Can you work these out from the model? Positions are in its coordinate system, mm. Face numbers are marked on the shaded views. A direction names the side the tool comes from. Coordinates: 2 decimals unless noted, no trailing zeros. Loops run counter-clockwise (first coordinate to the right, second up) from the corner with the lowest first, then second, coordinate; pieces in that order, holes last. Notation, with made-up numbers: (11.25, -24) -> (67.25, -24) arc R25 ccw to (67.25, 8) -> close; hole circle Ø1 at (-18.5, 48). An arc over 180 degrees is marked (long way). Use one line per item in the form item = value. Start each with the question number.
(1) Imagine slicing it at B-B (z = 385.5). List the corners of the cut face in (x, y) for me.
(2) I'm going to push flat-ended pins straight in: pin 1 (5 mm diameter, centred on x = 95.5, z = 207, fed in from -Y); pin 2 (5 mm diameter, centred on x = 414.5, y = -167, fed in from +Z); pin 3 (2 mm diameter, centred on y = -805, z = -1, fed in from -X). Where does each tip first touch, or does it pass through?
(3) Imagine slicing it at C-C (x = 127). List the corners of the cut face in (y, z) for me, plus the area to 3 significant figures.
(4) Imagine slicing it at D-D (x = 386). List the corners of the cut face in (y, z) for me, plus the area to 3 significant figures.
(5) I need wall thicknesses on line 1 (X direction, y = -793.5, z = 149); line 2 (Y direction, x = 472, z = 173); line 3 (Y direction, x = 45.5, z = 67.5). Which ranges of each line are inside material? Lowest first, please. Write a range as [from, to].
(6) On a 3-axis mill with a long thin cutter (end or side, diameter ignored), from which of +Z, -Z, +X, -X, +Y, -Y can I reach the whole of each face in a straight line? I mean the marked faces 5, 6 and 7. Say none if no direction works.
(7) Thinking about a two-plate mould opening in Y: for the marked faces 1, 2, 3 and 4, which applies, released by +Y, released by -Y, zero draft, split by the parting line, or undercut?
(8) Imagine slicing it at A-A (y = -231). List the corners of the cut face in (x, z) for me.
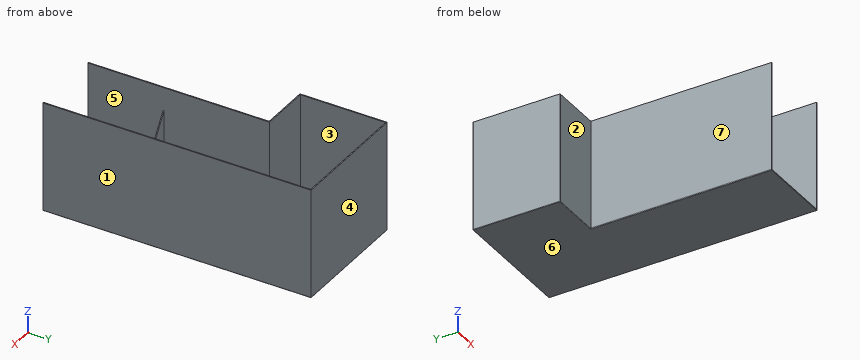
```python
from build123d import *

# Parameters (mm, degrees)
F1_DEPTH  = 426
F3_DEPTH  = 4
F4_R      = 2
F7_DEPTH  = 4
F8_DEPTH  = 4
F11_DEPTH = 4


# Not quite as in the source:
# - a feature names something its author has since deleted; it is built from what else it names


with BuildPart() as f1:
    # F0 (on Top) → F1 (new body)
    with BuildSketch(Plane.XY):
        Polygon((495, 0), (0, 0), (0, -343), (200, -343), (200, -1053), (204, -1053), (204, -339), (4, -339), (4, -4), (491, -4), (491, -1053), (495, -1053), align=None)
    extrude(amount=F1_DEPTH)

    # F2 (on Top) → F3 (join)
    with BuildSketch(Plane.XY):
        Polygon((0, -343), (200, -343), (199.9874711037, -1053), (495, -1053), (495, 0), (0, 0), align=None)
    extrude(amount=-F3_DEPTH)

    # F4
    f4_edges = [f1.edges().sort_by_distance(p)[0] for p in [
        (100, -343, -4),
        (0, -171.5, -4),
        (247.5, 0, -4),
        (0, -343, 211),
        (0, 0, 211),
        (495, 0, 211),
        (199.993736, -698, -4),
        (495, -526.5, -4),
    ]]
    fillet(f4_edges, radius=F4_R)

    # F6 (on offset) → F7 (join)
    with BuildSketch(Plane.XZ.offset(753)):
        Polygon((426, 0), (204, 335), (204, 0), align=None)
    extrude(amount=F7_DEPTH)

    # F6 (on offset) → F8 (join)
    with BuildSketch(Plane.XZ.offset(753)):
        Polygon((426, 0), (204, 335), (204, 0), align=None)
    extrude(amount=F8_DEPTH)

    # F10 (on offset) → F11 (join)
    with BuildSketch(Plane.XZ.offset(153)):
        Polygon((491, 335), (269, 0), (491, 0), align=None)
    extrude(amount=F11_DEPTH)


solid = f1.part
```
Worked out:
q1.outline = (0, -341) arc R2 ccw to (2, -343) -> (200, -343) -> (200, -1053) -> (204, -1053) -> (204, -339) -> (4, -339) -> (4, -4) -> (491, -4) -> (491, -1053) -> (495, -1053) -> (495, -2) arc R2 ccw to (493, 0) -> (2, 0) arc R2 ccw to (0, -2) -> close
q2.pin_1 = -343
q2.pin_2 = 0
q2.pin_3 = 199.99
q3.outline = (-343, -2) arc R2 ccw to (-341, -4) -> (-2, -4) arc R2 ccw to (0, -2) -> (0, 426) -> (-4, 426) -> (-4, 0) -> (-339, 0) -> (-339, 426) -> (-343, 426) -> close
q3.area = 4,780 mm2
q4.outline = (-1053, -4) -> (-2, -4) arc R2 ccw to (0, -2) -> (0, 426) -> (-4, 426) -> (-4, 0) -> (-153, 0) -> (-153, 176.55) -> (-157, 176.55) -> (-157, 0) -> (-753, 0) -> (-753, 60.36) -> (-757, 60.36) -> (-757, 0) -> (-1053, 0) -> close
q4.area = 6,860 mm2
q5.line_1 = [200, 204], [491, 495]
q5.line_2 = [-157, -153], [-4, 0]
q5.line_3 = [-343, -339], [-4, 0]
q6.face_5 = +Z
q6.face_6 = -Z, +X, -X, +Y, -Y
q6.face_7 = +Z, -Z, -X, -Y
q7.face_1 = zero draft
q7.face_2 = released by -Y
q7.face_3 = undercut
q7.face_4 = released by +Y
q8.outline = (0, -2) arc R2 ccw to (2, -4) -> (493, -4) arc R2 ccw to (495, -2) -> (495, 426) -> (491, 426) -> (491, 0) -> (4, 0) -> (4, 426) -> (0, 426) -> close
